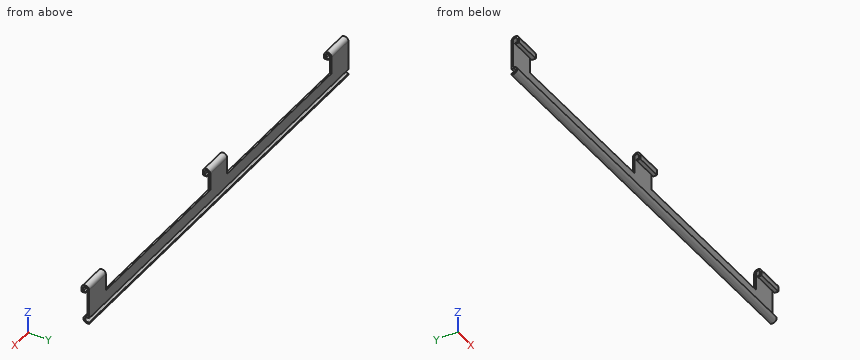
from build123d import *

# Parameters (mm, degrees)
F1_DEPTH      = 193.3
F2_W          = 155.8
F2_H          = 27.6261721705
F2_H_2        = 29.0520395572
F3_DEPTH      = 392
F3_DEPTH_BACK = 6.9075074824


# Not quite as in the source:
# - an extrude ends at something that could not be found from the text; its depth is read off the source's solid


with BuildPart() as f1:
    # F0 (on Right) → F1 (new body, symmetric)
    with BuildSketch(Plane.YZ):
        with BuildLine():
            Line((0, -17.0077651882), (0, -15.5077651882))
            Line((0, -15.5077651882), (-1.6385802936, -15.5077651882))
            ThreePointArc((-1.6385802936, -15.5077651882), (-3.6361192163, -13.605291718), (-1.8332301129, -11.5174320644))
            Line((-1.8332301129, -11.5174320644), (0, -11.5174320644))
            Line((0, -11.5174320644), (0, 15.5389810706))
            ThreePointArc((0, 15.5389810706), (-3.59937308, 18.9891420146), (-6.8941418337, 15.2470041272))
            Line((-6.8941418337, 15.2470041272), (-6.8941418337, 11.6459712901))
            Line((-6.8941418337, 11.6459712901), (-3.368163947, 11.6459712901))
            Line((-3.368163947, 11.6459712901), (-3.368163947, 12.6215412629))
            Line((-3.368163947, 12.6215412629), (-5.4103266448, 12.6215412629))
            Line((-5.4103266448, 12.6215412629), (-5.4103266448, 15.5389810706))
            ThreePointArc((-5.4103266448, 15.5389810706), (-3.5143862992, 17.4950989506), (-1.5, 15.661186523))
            Line((-1.5, 15.661186523), (-1.5, -10.0106816226))
            ThreePointArc((-1.5, -10.0106816226), (-5.1378081699, -13.4385473486), (-1.6385802936, -17.0077651882))
            Line((-1.6385802936, -17.0077651882), (0, -17.0077651882))
        make_face()
    extrude(amount=F1_DEPTH, both=True)

    # F2 (on Front) → F3 (cut, two sides)
    with BuildSketch(Plane.XZ) as f3_sk:
        with Locations((-90.4, 13.8130860853)):
            Rectangle(F2_W, F2_H)
        with Locations((90.4, 14.5260197786)):
            Rectangle(F2_W, F2_H_2)
    extrude(amount=-F3_DEPTH, mode=Mode.SUBTRACT)
    extrude(f3_sk.sketch, amount=F3_DEPTH_BACK, mode=Mode.SUBTRACT)


solid = f1.part
CAD build for the part. Positions are in the model's coordinates, mm. Round coordinates to 2 decimals unless told otherwise and drop trailing zeros. Write each loop counter-clockwise with the first axis right and the second up, starting at its lowest first coordinate (ties: lowest second). Pieces come first, ordered by that corner, then holes.
(1) Probe line 1 along X through (y, z) = (-1.25, 7); line 2 along Z through (x, y) = (144, -2); line 3 along Z through (x, y) = (-111, -0.75). List the from-to ranges inside material, lowest first.
(2) Slice it at A-A, the plane z = 5.5. Write the cut outline in (x, y), and give its area (4 significant figures).
(3) Drop flat-ended pins along their axis: P1, Ø4, axis at x = -29.5, y = -2.5, coming from the +Z side; P2, Ø1, axis at x = 4, y = -4.5, coming from the +Z side; P3, Ø6, axis at x = -125.5, z = -4.5, coming from the -Y side; P4, Ø2, axis at x = 15, z = 9, coming from the -Y side. Give the stop position or say it passes through.
(4) Slice it at B-B, the plane x = 21.5. Write the cut outline in (y, z).
From the geometry:
1. line 1: x = -193.3 to -168.3, -12.5 to 12.5, 168.3 to 193.3
1. line 2: z = -16.99 to -15.47, -11.54 to -10.03
1. line 3: z = -17.01 to -15.51, -11.52 to 0
2. outline: (-193.3, -1.5) - (-168.3, -1.5) - (-168.3, 0) - (-193.3, 0) - close; (-12.5, -1.5) - (12.5, -1.5) - (12.5, 0) - (-12.5, 0) - close; (168.3, -1.5) - (193.3, -1.5) - (193.3, 0) - (168.3, 0) - close
2. area: 112.5 mm2
3. P1: stops at z = 0
3. P2: stops at z = 18.95
3. P3: stops at y = -1.5
3. P4: passes through
4. outline: (-1.83, -11.52) - (0, -11.52) - (0, 0) - (-1.5, 0) - (-1.5, -10.01) arc R3.5 ccw (long way) to (-1.64, -17.01) - (0, -17.01) - (0, -15.51) - (-1.64, -15.51) arc R2 cw to start
